Build history of the part. All positions in model axes, mm. A direction names the side the tool comes from. Round coordinates to 2 decimals unless told otherwise and drop trailing zeros. Write each loop counter-clockwise with the first axis right and the second up, starting at its lowest first coordinate (ties: lowest second). Pieces come first, ordered by that corner, then holes. Notation, with made-up numbers: M -35,36 L -12,36 A30 cw -12,59 Z; hole C 67,-14.75 d11. An arc over 180 degrees is marked long. Use a Markdown table: item, result.
from build123d import *

# Parameters (mm, degrees)
BOSS_EXTRUDE1_DEPTH = 4
SKETCH2_W           = 162.38
SKETCH2_H           = 120.39
SKETCH2_W_2         = 157.38
SKETCH2_H_2         = 116.682954798
BOSS_EXTRUDE2_DEPTH = 10
FILLET1_R           = 10
FILLET2_R           = 5
SKETCH3_R           = 2
CUT_EXTRUDE1_DEPTH  = 182
SKETCH4_R           = 2
CUT_EXTRUDE2_DEPTH  = 182


with BuildPart() as part:
    # Sketch1 → Boss-Extrude1 (new body)
    with BuildSketch(Plane(origin=(0, 0, 0), x_dir=(1, 0, 0), z_dir=(0, 1, 0))):
        Polygon((-84.19, 63.195), (84.19, 63.195), (84.19, 10), (104.19, 10), (104.19, -10), (84.19, -10), (84.19, -63.195), (-84.19, -63.195), (-84.19, -10), (-104.19, -10), (-104.19, 10), (-84.19, 10), align=None)
    extrude(amount=BOSS_EXTRUDE1_DEPTH)

    # Sketch2 → Boss-Extrude2 (add)
    with BuildSketch(Plane(origin=(0, 4, 0), x_dir=(1, 0, 0), z_dir=(0, 1, 0))):
        Rectangle(SKETCH2_W, SKETCH2_H)
        Rectangle(SKETCH2_W_2, SKETCH2_H_2, mode=Mode.SUBTRACT)
    extrude(amount=BOSS_EXTRUDE2_DEPTH)

    # Fillet1
    fillet1_edges = [part.edges().sort_by_distance(p)[0] for p in [
        (104.19, 2, -10),
        (104.19, 2, 10),
        (-104.19, 2, -10),
        (-104.19, 2, 10),
    ]]
    fillet(fillet1_edges, radius=FILLET1_R - 0.0001)  # a hair under: the kernel refuses the full size

    # Fillet2
    fillet2_edges = [part.edges().sort_by_distance(p)[0] for p in [
        (84.19, 2, 63.195),
        (-84.19, 2, 63.195),
        (-84.19, 2, -63.195),
        (84.19, 2, -63.195),
    ]]
    fillet(fillet2_edges, radius=FILLET2_R)

    # Sketch3 → Cut-Extrude1 (cut)
    with BuildSketch(Plane(origin=(81.19, 0, 0), x_dir=(0, 0, -1), z_dir=(1, 0, 0))):
        with Locations((0, 9)):
            Circle(SKETCH3_R)
    extrude(amount=-CUT_EXTRUDE1_DEPTH, mode=Mode.SUBTRACT)

    # Sketch4 → Cut-Extrude2 (cut)
    with BuildSketch(Plane(origin=(0, 0, -63.195), x_dir=(-1, 0, 0), z_dir=(0, 0, -1))):
        with Locations((39.19, 9)):
            Circle(SKETCH4_R)
        with Locations((-39.19, 9)):
            Circle(SKETCH4_R)
    extrude(amount=-CUT_EXTRUDE2_DEPTH, mode=Mode.SUBTRACT)


solid = part.part
Q1. Drop flat-ended pins along their axis: P1, Ø4.5, axis at y = 3, z = 40.5, coming from the +X side; P2, Ø1.5, axis at x = 53, z = -43.5, coming from the +Y side; P3, Ø3, axis at x = 3, y = 6.5, coming from the +Z side (3 decimals); P4, Ø10, axis at x = -11, z = 32, coming from the -Y side. Give the stop position or say it passes through.
Response values:
| item | result |
|---|---|
| P1 | stops at x = 84.19 |
| P2 | stops at y = 4 |
| P3 | stops at z = 60.195 |
| P4 | stops at y = 0 |
Q2. Which spindle directions (+Z, -Z, +X, -X, +Y, -Y) get a long thin tool onto all of the face, cutting with end or side? Do faces 4 (the flat face through (-89, 2, 10)), 5 (the flat face through (-81.19, 11, 1)), 6 (the flat face through (-1, 9, 58.341)). Say none if no direction does.
Response values:
| item | result |
|---|---|
| face 4 | +Z, -X, +Y, -Y |
| face 5 | +Z, -Z, -X, +Y |
| face 6 | +Y |
Q3. Two-plate mould, pull along Y, no slides. Class faces 1 (the flat face through (1, 4, -1)), 2 (the cylindrical face through (41.188, 9.088, 59.255)), 3 (the flat face through (89, 2, -10)): +Y half, -Y half, draft (parallel to the pull), parting line (faces both ways), or undercut.
Response values:
| item | result |
|---|---|
| face 1 | +Y half |
| face 2 | undercut |
| face 3 | draft |
Q4. Cut at D-D on x = -74. Give the cut face in (y, z) (3 decimals).
Response values:
| item | result |
|---|---|
| outline | M 0,-63.195 L 4,-63.195 L 4,-60.195 L 14,-60.195 L 14,-58.341 L 4,-58.341 L 4,58.341 L 14,58.341 L 14,60.195 L 4,60.195 L 4,63.195 L 0,63.195 Z |
Q5. Cut at B-B on y = 9. Count the separate pieces of the cut face and the enclosed holes in it, and give its area (3 significant figures).
Response values:
| item | result |
|---|---|
| separate pieces | 6 |
| enclosed holes | 0 |
| area | 1,140 mm2 |
Q6. Drill centre lines: L1, parallel to Y at x = -39, z = -59; L2, parallel to Z at x = -74, y = 13.5 (3 decimals); L3, parallel to X at y = 7, z = -4.5. Where is each one in solid material? Low to high.
Response values:
| item | result |
|---|---|
| L1 | y = 0 to 7.01, 10.99 to 14 |
| L2 | z = -60.195 to -58.341, 58.341 to 60.195 |
| L3 | x = -81.19 to -78.69, 78.69 to 81.19 |
Q7. Cut at C-C on z = 16.5. Give the cut face in (x, y).
Response values:
| item | result |
|---|---|
| outline | M -84.19,0 L 84.19,0 L 84.19,4 L 81.19,4 L 81.19,14 L 78.69,14 L 78.69,4 L -78.69,4 L -78.69,14 L -81.19,14 L -81.19,4 L -84.19,4 Z |
Q8. Cut at A-A on x = 39.19. Give the cut face in (y, z) (3 decimals), and give its area (3 significant figures).
Response values:
| item | result |
|---|---|
| outline | M 0,-63.195 L 4,-63.195 L 4,-60.195 L 7,-60.195 L 7,-58.341 L 4,-58.341 L 4,58.341 L 7,58.341 L 7,60.195 L 4,60.195 L 4,63.195 L 0,63.195 Z; M 11,-60.195 L 14,-60.195 L 14,-58.341 L 11,-58.341 Z; M 11,58.341 L 14,58.341 L 14,60.195 L 11,60.195 Z |
| area | 528 mm2 |
